```python
from build123d import *

# Parameters (mm, degrees)
F0_W     = 1676.4
F0_H     = 50.8
F1_DEPTH = 6.35
F2_W     = 25.4
F2_H     = 25.4
F3_DEPTH = 254


with BuildPart() as f1:
    # F0 (on Front) → F1 (new body)
    with BuildSketch(Plane.XZ):
        Rectangle(F0_W, F0_H)
    extrude(amount=F1_DEPTH)

    # F2 (on face) → F3 (join)
    with BuildSketch(Plane.XZ.offset(6.35)):
        with Locations((-774.7, -12.7)):
            Rectangle(F2_W, F2_H)
        with Locations((774.7, -12.7)):
            Rectangle(F2_W, F2_H)
        Polygon((-12.7, 0), (-12.7, -25.4), (0, -25.4), (12.7, -25.4), (12.7, 0), (0, 0), align=None)
    extrude(amount=F3_DEPTH)


solid = f1.part
```
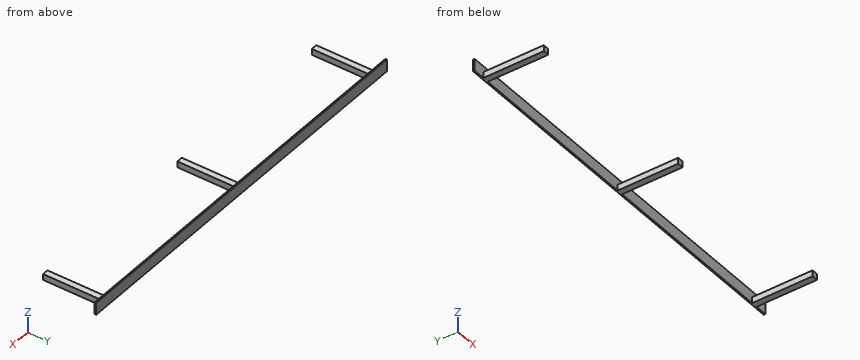
CAD build for the part. Positions are in the model's coordinates, mm. Round coordinates to 2 decimals unless told otherwise and drop trailing zeros. Loops run counter-clockwise (first coordinate to the right, second up) from the corner with the lowest first, then second, coordinate; pieces in that order, holes last. Notation, with made-up numbers: M 74,-39.5 L 94,-39.5 A9 cw 94,-29.5 Z; hole C 88,-1.75 d3. An arc over 180 degrees is marked long. Use a Markdown table: item, result. Add a question column.
(1) Flat gauge pins, fed straight in: pin 1 (6 mm diameter, centred on x = 141.5, z = -12, fed in from -Y); pin 2 (20.5 mm diameter, centred on y = -193, z = -12.5, fed in from +X); pin 3 (5 mm diameter, centred on y = -34.5, z = -19, fed in from -X). Where does each tip first touch, or does it go through?
(2) Cut at B-B (z = -17). Give the cut face in (x, y).
(3) Cut at C-C (x = -200.5). Give the cut face in (y, z).
(4) Drill centre lines: line 1 (X direction, y = -57.5, z = -16); line 2 (Y direction, x = -243.5, z = 10). Where is each one in solid material? Low to high.
(5) Cut at A-A (y = -228). Give the cut face in (x, z), and give its area (3 significant figures).
Geometry says:
| question | item | result |
|---|---|---|
| 1 | pin 1 | stops at y = -6.35 |
| 1 | pin 2 | stops at x = 787.4 |
| 1 | pin 3 | stops at x = -787.4 |
| 2 | outline | M -838.2,-6.35 L -787.4,-6.35 L -787.4,-260.35 L -762,-260.35 L -762,-6.35 L -12.7,-6.35 L -12.7,-260.35 L 12.7,-260.35 L 12.7,-6.35 L 762,-6.35 L 762,-260.35 L 787.4,-260.35 L 787.4,-6.35 L 838.2,-6.35 L 838.2,0 L -838.2,0 Z |
| 3 | outline | M -6.35,-25.4 L 0,-25.4 L 0,25.4 L -6.35,25.4 Z |
| 4 | line 1 | x = -787.4 to -762, -12.7 to 12.7, 762 to 787.4 |
| 4 | line 2 | y = -6.35 to 0 |
| 5 | outline | M -787.4,-25.4 L -762,-25.4 L -762,0 L -787.4,0 Z; M -12.7,-25.4 L 12.7,-25.4 L 12.7,0 L -12.7,0 Z; M 762,-25.4 L 787.4,-25.4 L 787.4,0 L 762,0 Z |
| 5 | area | 1,940 mm² |
